Read the model definition and answer for the solid it produces. Units are mm, in the model's axes. A direction names the side the tool comes from. Coordinates: 2 decimals unless noted, no trailing zeros. Loops run counter-clockwise (first coordinate to the right, second up) from the corner with the lowest first, then second, coordinate; pieces in that order, holes last.
from build123d import *

# Parameters (mm, degrees)
SKETCH1_W           = 20
SKETCH1_H           = 30
BOSS_EXTRUDE1_DEPTH = 2
SKETCH2_R           = 3
CUT_EXTRUDE1_DEPTH  = 2
SKETCH4_W           = 2
SKETCH4_H           = 2.5
CUT_EXTRUDE2_DEPTH  = 32.685959036
BOSS_EXTRUDE2_DEPTH = 30
BOSS_EXTRUDE3_START = 3
SKETCH6_R           = 5
SKETCH6_R_2         = 3
BOSS_EXTRUDE3_DEPTH = 3
BOSS_EXTRUDE4_DEPTH = 2
SKETCH8_W           = 14
SKETCH8_H           = 28
BOSS_EXTRUDE5_DEPTH = 2
SKETCH9_R           = 9.691307823
SKETCH9_R_2         = 8.81055964
BOSS_EXTRUDE6_DEPTH = 4
BOSS_EXTRUDE7_DEPTH = 30
CUT_EXTRUDE3_DEPTH  = 41.577802203
BOSS_EXTRUDE8_DEPTH = 13.3
SKETCH17_W          = 10
SKETCH17_H          = 5
CUT_EXTRUDE5_DEPTH  = 2


with BuildPart() as part:
    # Sketch1 → Boss-Extrude1 (new body)
    with BuildSketch(Plane(origin=(0, 0, 0), x_dir=(0, 0, -1), z_dir=(1, 0, 0))):
        Rectangle(SKETCH1_W, SKETCH1_H)
    extrude(amount=BOSS_EXTRUDE1_DEPTH)

    # Sketch2 → Cut-Extrude1 (cut)
    with BuildSketch(Plane.ZY):
        Circle(SKETCH2_R)
    extrude(amount=-CUT_EXTRUDE1_DEPTH, mode=Mode.SUBTRACT)

    # Sketch4 → Cut-Extrude2 (cut, through all)
    with BuildSketch(Plane(origin=(0, 15, 0), x_dir=(1, 0, 0), z_dir=(0, 1, 0))):
        with Locations((1, 8.75)):
            Rectangle(SKETCH4_W, SKETCH4_H)
        with Locations((1, -8.75)):
            Rectangle(SKETCH4_W, SKETCH4_H)
    extrude(amount=-CUT_EXTRUDE2_DEPTH, mode=Mode.SUBTRACT)

    # Sketch5 → Boss-Extrude2 (add, through all)
    with BuildSketch(Plane(origin=(0, 15, 0), x_dir=(1, 0, 0), z_dir=(0, 1, 0))):
        Polygon((2, 7.5), (-6.625791341, 14), (-9.949071623, 14), (0, 6.502836784), align=None)
        Polygon((-6.625791341, -14), (-9.949071623, -14), (0, -6.502836784), (2, -7.5), align=None)
    extrude(amount=-BOSS_EXTRUDE2_DEPTH)

    # Sketch6 → Boss-Extrude3 (add)
    with BuildSketch(Plane.ZY.offset(BOSS_EXTRUDE3_START)):
        with Locations(Location((0, 0, 0), (0, 0, 180))):
            Circle(SKETCH6_R)
        Circle(SKETCH6_R_2, mode=Mode.SUBTRACT)
    extrude(amount=-BOSS_EXTRUDE3_DEPTH)

    # Sketch7 → Boss-Extrude4 (add)
    with BuildSketch(Plane.XZ.offset(15)):
        Polygon((-9.949071623, 14), (-6.625791341, 14), (2, 7.5), (2, -7.5), (-6.625791341, -14), (-9.949071623, -14), align=None)
    extrude(amount=BOSS_EXTRUDE4_DEPTH)

    # Sketch8 → Boss-Extrude5 (add)
    with BuildSketch(Plane.XZ.offset(17)):
        with Locations((-16.949071623, 0)):
            Rectangle(SKETCH8_W, SKETCH8_H)
    extrude(amount=-BOSS_EXTRUDE5_DEPTH)

    # Sketch9 → Boss-Extrude6 (add)
    with BuildSketch(Plane(origin=(0, -15, 0), x_dir=(1, 0, 0), z_dir=(0, 1, 0))):
        with Locations(Location((-13.884110901, 4.279502294, 0), (0, 0, 90))):
            Circle(SKETCH9_R)
        with Locations(Location((-13.884110901, 4.279502294, 0), (0, 0, 270))):
            Circle(SKETCH9_R_2, mode=Mode.SUBTRACT)
    extrude(amount=BOSS_EXTRUDE6_DEPTH)

    # Sketch10 → Boss-Extrude7 (add)
    with BuildSketch(Plane(origin=(0, -15, 0), x_dir=(1, 0, 0), z_dir=(0, 1, 0))):
        Polygon((-6.625791341, -14), (-6.625791341, -13), (-7.754589709, -13), (-22.949071623, -13), (-22.949071623, 13.1), (-7.754589709, 13.1), (-6.625791341, 13.1), (-6.625791341, 14), (-23.949071623, 14), (-23.949071623, -14), align=None)
    extrude(amount=BOSS_EXTRUDE7_DEPTH)

    # Sketch11 → Cut-Extrude3 (cut, through all)
    with BuildSketch(Plane(origin=(0, 0, -14), x_dir=(-1, 0, 0), z_dir=(0, 0, -1))):
        Polygon((16.934110901, 1.7), (23.949071623, 1.7), (23.949071623, 15), (6.625791341, 15), (6.625791341, 1.7), align=None)
    extrude(amount=-CUT_EXTRUDE3_DEPTH, mode=Mode.SUBTRACT)

    # Sketch13 → Boss-Extrude8 (add)
    with BuildSketch(Plane(origin=(0, 1.7, 0), x_dir=(1, 0, 0), z_dir=(0, 1, 0))):
        Polygon((-6.625791341, -14), (-6.625791341, -6.502836784), (0, -6.502836784), (0, -9.0071081), align=None)
        Polygon((0, 9.0071081), (-6.625791341, 14), (-6.625791341, 6.502836784), (0, 6.502836784), align=None)
    extrude(amount=BOSS_EXTRUDE8_DEPTH)

    # Sketch17 → Cut-Extrude5 (cut)
    with BuildSketch(Plane.XZ.offset(17)):
        with Locations((-14.949071623, 9.5)):
            Rectangle(SKETCH17_W, SKETCH17_H)
    extrude(amount=-CUT_EXTRUDE5_DEPTH, mode=Mode.SUBTRACT)


solid = part.part
Q1. Straight lines are drawn through the part: probe 1 along X at (y, z) = (-10, -2); probe 2 along Z at (x, y) = (-16.75, -0.5); probe 3 along Z at (x, y) = (-14.75, -14.5). For each, find the intervals that lie inside material, in ascending order.
Findings below:
probe 1: x = -23.95 to -22.95, 0 to 2
probe 2: z = -14 to -13.1, 13 to 14
probe 3: z = -14 to -13.05, 4.49 to 5.37, 13 to 14
Q2. A cutting plane is placed at C-C (z = 0). Give the vertices of the cut face in (x, y).
Findings below:
outline: (-23.95, -17) - (2, -17) - (2, -3) - (-3, -3) - (-3, -5) - (0, -5) - (0, -15) - (-5.19, -15) - (-5.19, -11) - (-6.18, -11) - (-6.18, -15) - (-21.59, -15) - (-21.59, -11) - (-22.58, -11) - (-22.58, -15) - (-22.95, -15) - (-22.95, 1.7) - (-23.95, 1.7) - close; (-3, 3) - (2, 3) - (2, 15) - (0, 15) - (0, 5) - (-3, 5) - close
Q3. A cutting plane is placed at A-A (y = -10). Give the vertices of the cut face in (x, z), then the cut area to 3 significant figures.
Findings below:
outline: (-23.95, -14) - (-6.63, -14) - (2, -7.5) - (2, 7.5) - (-6.63, 14) - (-23.95, 14) - close; hole (-22.95, -13.1) - (-8.75, -13.1) - (0, -6.5) - (0, 6.5) - (-8.62, 13) - (-22.95, 13) - close
area: 128 mm2
Q4. A cutting plane is placed at B-B (x = -15.5). Give the vertices of the cut face in (y, z), then the cut area to 3 significant figures.
Findings below:
outline: (-17, -14) - (1.7, -14) - (1.7, -13.1) - (-11, -13.1) - (-11, -12.94) - (-15, -12.94) - (-15, 4.38) - (-11, 4.38) - (-11, 5.28) - (-15, 5.28) - (-15, 7) - (-17, 7) - close; (-17, 12) - (-15, 12) - (-15, 13) - (1.7, 13) - (1.7, 14) - (-17, 14) - close
area: 81.9 mm2
Q5. Flat-ended cylindrical pins translate along their axes: pin 1 Ø1.5 at (x, z) = (-20.5, -10.5) entering from +Y; pin 2 Ø8 at (x, y) = (-4, 6.5) entering from +Z; pin 3 Ø10.5 at (x, z) = (-13.88, -4.28) entering from +Y. Find the tip coordinate at first contact, or state that the pin passes through.
Findings below:
pin 1: stops at y = -11
pin 2: stops at z = 14
pin 3: stops at y = -15
Q6. Determine the mould class of faces 5 (the face through (-5, 1.7, -8)), 6 (the face through (-15, -8, 14)), 7 (the face through (-6.626, 8, -10)), 8 (the face through (-15, -16, 12)) for opening direction X: +X half, -X half, draft (parallel to the pull), parting line (faces both ways), or undercut.
Findings below:
face 5: undercut
face 6: draft
face 7: -X half
face 8: undercut
Q7. A cutting plane is placed at D-D (y = 0). Give the vertices of the cut face in (x, z), then the cut area to 3 significant figures.
Findings below:
outline: (-23.95, -14) - (-6.63, -14) - (2, -7.5) - (2, -3) - (-3, -3) - (-3, -5) - (0, -5) - (0, -6.5) - (-8.75, -13.1) - (-22.95, -13.1) - (-22.95, 13) - (-8.62, 13) - (0, 6.5) - (0, 5) - (-3, 5) - (-3, 3) - (2, 3) - (2, 7.5) - (-6.63, 14) - (-23.95, 14) - close
area: 128 mm2
Q8. Which of the six approach directions +Z, -Z, +X, -X, +Y, -Y give full straight-line access (tool end or side, diameter ignored) to faces 1 (the face through (-3, 8, -6.503)), 2 (the face through (-19.949, -16, 9)), 3 (the face through (-1, 0, -3)), 4 (the face through (-3, 3.3, 0.1))?
Findings below:
face 1: -X, +Y
face 2: +Y, -Y
face 3: +X
face 4: +Y
